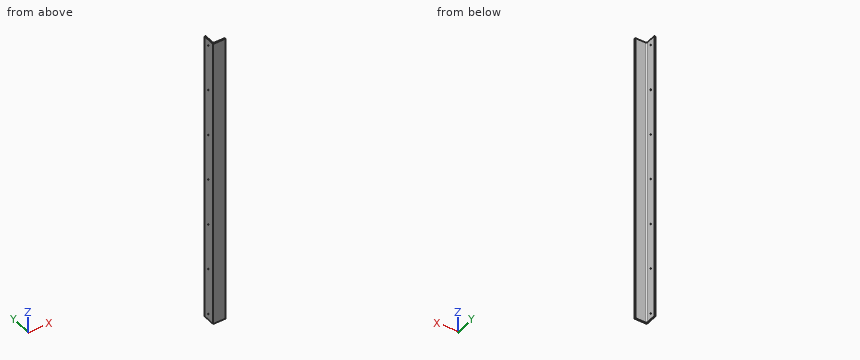
from build123d import *

# Parameters (mm, degrees)
BOSS_EXTRUDE1_DEPTH             = 1828.8
F_0_25_6_74688_DIAMETER_HOLE1_D = 6.74688


with BuildPart() as part:
    # Sketch1 → Boss-Extrude1 (new body)
    with BuildSketch(Plane.XY):
        with BuildLine():
            Line((0, 0), (0, 76.2))
            Line((0, 76.2), (6.35, 76.2))
            Line((6.35, 76.2), (6.35, 12.7))
            ThreePointArc((6.35, 12.7), (8.209871939, 8.209871939), (12.7, 6.35))
            Line((12.7, 6.35), (76.2, 6.35))
            Line((76.2, 6.35), (76.2, 0))
            Line((76.2, 0), (0, 0))
        make_face()
    extrude(amount=BOSS_EXTRUDE1_DEPTH)

    # Ø0.25 (6.74688) Diameter Hole1 (through all)
    with Locations(Plane(origin=(6.35, 0, 0), x_dir=(0, 0, -1), z_dir=(1, 0, 0))):
        with Locations((-1790.7, 44.45), (-1498.6, 44.45), (-1206.5, 44.45), (-914.4, 44.45), (-622.3, 44.45), (-330.2, 44.45), (-38.1, 44.45)):
            Hole(F_0_25_6_74688_DIAMETER_HOLE1_D / 2)


solid = part.part
Verification items for the finished model (mm, model axes). Give positions to 0.01 mm unless a question says otherwise; leave off trailing zeros. Loops run counter-clockwise (first coordinate to the right, second up) from the corner with the lowest first, then second, coordinate; pieces in that order, holes last.
1) Sectioned sample at A-A, the plane z = 310.5. Enter the section's corners in (x, y).
2) Thickness scan on line 1 along Y through (x, z) = (1.75, 622.3); line 2 along X through (y, z) = (60, 1108.5). Record the ranges inside material, lowest first.
3) Depth check by flat-ended pin: pin 1 Ø4 at (y, z) = (42.5, 1164.5) entering from -X; pin 2 Ø11 at (y, z) = (44.45, 1790.7) entering from +X; pin 3 Ø19 at (x, z) = (58.5, 619) entering from +Y. Enter the tip coordinate at first touch or a pass-through.
4) Sectioned sample at B-B, the plane y = 27.5. Enter the section's corners in (x, z).
Answers:
1. outline: (0, 0) - (76.2, 0) - (76.2, 6.35) - (12.7, 6.35) arc R6.35 cw to (6.35, 12.7) - (6.35, 76.2) - (0, 76.2) - close
2. line 1: y = 0 to 41.08, 47.82 to 76.2
2. line 2: x = 0 to 6.35
3. pin 1: stops at x = 0
3. pin 2: stops at x = 6.35
3. pin 3: stops at y = 6.35
4. outline: (0, 0) - (6.35, 0) - (6.35, 1828.8) - (0, 1828.8) - close
